Autodesk Inventor part; units mm, degrees
ref_plane "YZ Plane" through (0, 0, 0) normal (1, 0, 0) x (0, 1, 0)
ref_plane "XZ Plane" through (0, 0, 0) normal (0, 1, 0) x (-1, 0, 0)
ref_plane "XY Plane" through (0, 0, 0) normal (0, 0, 1) x (1, 0, 0)
sketch "Sketch1" plane through (0, 0, 0) normal (0, 1, 0) x (-1, 0, 0)
  circle A0 centre (0, 0) radius 12.7
  dimension "d0" = 25.4
extrude "Extrusion1" add sketch "Sketch1" along normal blind 180
sketch "Sketch3" plane through (0, 180, 0) normal (0, 1, 0) x (1, 0, 0)
  point P0 (0, 0)
  point P1 (0, 0)
hole "Hole2" at (0, 180, 0) direction (0, -1, 0) diameter 10 end through all
sketch "Sketch4" plane through (0, 180, 0) normal (0, 1, 0) x (1, 0, 0)
  point P0 (0, 0)
  point P1 (0, -8.25)
  point P2 (-8.25, 0)
  point P3 (0, 8.25)
  point P4 (8.25, 0)
  dimension "d17" = 8.25
  dimension "d20" = 360
hole "Hole3" at (0, 180, 8.25) at (-8.25, 180, 0) at (0, 180, -8.25) at (8.25, 180, 0) direction (0, -1, 0) diameter 3 depth 38.1 tip angle 118
thread "Thread1"
thread "Thread2"
thread "Thread3"
thread "Thread4"
properties part number "BarraSolidaMotor"
Could you check a few things on this model? Use its own coordinates, in mm. A direction names the side the tool comes from. Round coordinates to 2 decimals unless told otherwise and drop trailing zeros. Loops run counter-clockwise (first coordinate to the right, second up) from the corner with the lowest first, then second, coordinate; pieces in that order, holes last. Notation, with made-up numbers: (13, -2.5) -> (19, -2.5) arc R22 cw to (19, 8.5) -> close; hole circle Ø3 at (-31.75, 15.5). An arc over 180 degrees is marked (long way). Use CSV: the item, a comma, the result in double quotes.
(1) For faces 1 (the cylindrical face through (-0.07, 160.68, -9.75)), 2 (the flat face through (-5.5, 180, 0.2)), which set-ups out of +Z, -Z, +X, -X, +Y, -Y let a thin tool reach every point of the face, with its end or its side?
Return value:
face 1,"+Y"
face 2,"+Z, -Z, +X, -X, +Y"
(2) If I drill on probe 1 along Z at (x, y) = (0, 142); probe 2 along X at (y, z) = (27, -3.5); probe 3 along Z at (x, y) = (3, 59), over which ranges is the centre line in solid material (lowest first)? Write a range as [from, to].
Return value:
probe 1,"z = [-12.7, -9.75], [-6.75, -5], [5, 6.75], [9.75, 12.7]"
probe 2,"x = [-12.21, -3.57], [3.57, 12.21]"
probe 3,"z = [-12.34, -4], [4, 12.34]"
(3) Suppose I cut it at B-B on y = 108. Write out the boundary of the cut face in (x, z), plus the area to 3 significant figures.
Return value:
outline,"circle Ø25.4 at (0, 0); hole circle Ø10 at (0, 0)"
area,"428 mm²"
(4) Will these pins go through, and if not, where does the flat tip stop? pin 1 Ø3 at (y, z) = (58, -9.5) entering from +X; pin 2 Ø1 at (x, y) = (8, 22) entering from -Z; pin 3 Ø3 at (x, y) = (-3.5, 24.5) entering from -Z.
Return value:
pin 1,"stops at x = 9.86"
pin 2,"stops at z = -10.25"
pin 3,"stops at z = -12.54"
(5) If we mould it in two halves opening along Z, with no side actions, what happens to faces 3 (the conical face through (-0.1, 141.155, -8.009)), 4 (the cylindrical face through (2.75, 88.74, 12.4)), 5 (the flat face through (-5.5, 0, 0.2))? For each: +Z half, -Z half, draft (parallel to the pull), parting line (faces both ways), or undercut.
Return value:
face 3,"undercut"
face 4,"parting line"
face 5,"draft"
(6) Suppose I cut it at A-A on z = 3. Write out the boundary of the cut face in (x, y).
Return value:
outline,"(-12.34, 0) -> (-4, 0) -> (-4, 180) -> (-12.34, 180) -> close; (4, 0) -> (12.34, 0) -> (12.34, 180) -> (4, 180) -> close"
